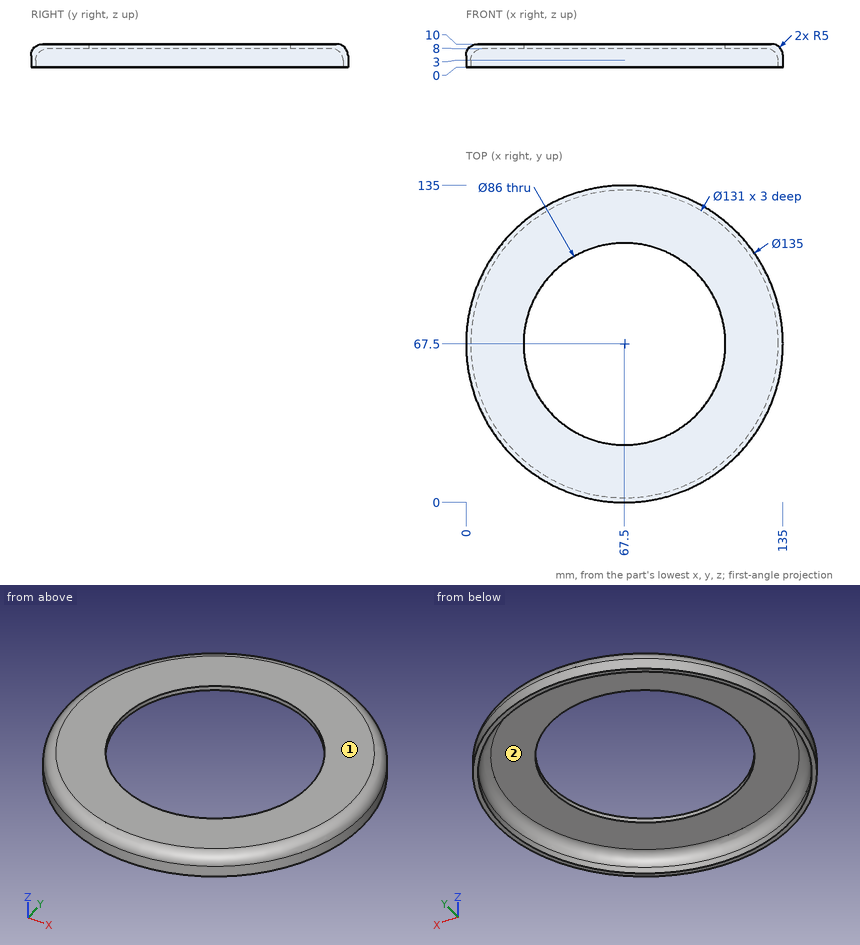
Answer from the drawing. Dimensions are ordinates in mm from the lowest x, y and z of the part. Coordinates: 2 decimals unless noted, no trailing zeros. Answer as CSV lines item,"result".
Q1. Find the intervals of material crossed by probe 1 along Z at (x, y) = (116.5, 60.5); probe 2 along Y at (x, z) = (67.5, 1.45); probe 3 along Y at (x, z) = (67.5, 8.85), in increasing order.
Findings:
probe 1,"z = 8 to 10"
probe 2,"y = 0 to 2, 133 to 135"
probe 3,"y = 1.81 to 24.5, 110.5 to 133.19"
Q2. For a pull along Y with two mould halves and no side action, classify the marked faces 1 and 2 as +Y half, -Y half, draft (parallel to the pull), parting line (faces both ways), or undercut.
Findings:
face 1,"draft"
face 2,"undercut"
Q3. Each of these flat-tipped pins is pushed along its axis until it touches: pin 1 (3 mm diameter, centred on y = 57, z = 4.5, fed in from -X); pin 2 (5 mm diameter, centred on x = 119, z = 7.5, fed in from +Y); pin 3 (3 mm diameter, centred on y = 84, z = 7.5, fed in from +X). Where does it stop, or does it pass through?
Findings:
pin 1,"stops at x = 0.6"
pin 2,"stops at y = 113.37"
pin 3,"stops at x = 133"
